Source: CAD feature listing. Evaluate the final solid. Frame: model axes, mm. A direction names the side the tool comes from. Coordinates: 2 decimals unless noted, no trailing zeros. Write each loop counter-clockwise with the first axis right and the second up, starting at its lowest first coordinate (ties: lowest second). Pieces come first, ordered by that corner, then holes. Notation, with made-up numbers: M 20.25,8.5 L 41.25,8.5 A28 ccw 41.25,44.5 Z; hole C 62,-22.5 d6. An arc over 180 degrees is marked long. One line per item, written item: value. Start each with the question number.
Item 1: Cut plane C-C, the plane y = 20. Output: boundary loops of the cut face in (x, z).
Item 2: Set-up query: faces 5 (the flat face through (2.6, 5, 4.9)), 6 (the flat face through (35, 15, 5)), 7 (the cylindrical face through (22.3, 22.5, 5.1)). Return all of +Z, -Z, +X, -X, +Y, -Y with unobstructed straight access to the full face (end or side cutting, diameter ignored); none if empty.
Item 3: Cut plane D-D, the plane x = 26.5. Output: boundary loops of the cut face in (y, z).
Item 4: Mould query, pull axis Z, two halves, no side actions, for faces 1 (the flat face through (10, 16, 5)), 2 (the flat face through (22, 10, 0)), 3 (the cylindrical face through (7, 3, 5)), 4 (the flat face through (22, 10, 10)). Classes: released by +Z, released by -Z, zero draft, split by the parting line, or undercut.
Item 5: Cut plane B-B, the plane z = 5. Output: boundary loops of the cut face in (x, y), then the cut area to 3 significant figures.
Item 6: Ray query, L1, parallel to X at y = 4.5, z = 5.25; L2, parallel to Z at x = 40, y = 1.15; L3, parallel to Y at x = 42, z = 4.25. Return the intervals inside material, ascending. Write a range as from..to.
Item 7: Cut plane A-A, the plane x = 5. Output: boundary loops of the cut face in (y, z).
Item 8: Pin query (flat end, axial travel): P1, Ø4.5, axis at x = 3.5, z = 6.5, coming from the +Y side; P2, Ø2.5, axis at x = 5, z = 5, coming from the +Y side; P3, Ø6, axis at y = 10, z = 6, coming from the -X side. Return the tip coordinate at first contact, or that it passes through.
```python
from build123d import *

# Parameters (mm, degrees)
F1_DEPTH = 10
F3_D     = 5
F5_D     = 4
F6_R     = 0.5
F7_R     = 1


with BuildPart() as f1:
    # F0 (on Top) → F1 (new body)
    with BuildSketch(Plane.XY):
        Polygon((0, 5), (0, 0), (45, 0), (45, 5), (35, 5), (35, 25), (10, 25), (10, 5), align=None)
    extrude(amount=F1_DEPTH)

    # F3 (through all)
    with Locations(Plane.YZ.offset(35)):
        with Locations((20, 5)):
            Hole(F3_D / 2)

    # F5 (through all)
    with Locations(Plane.XZ):
        with Locations((5, 5), (40, 5)):
            Hole(F5_D / 2)

    # F6
    f6_edges = [f1.edges().sort_by_distance(p)[0] for p in [
        (0, 2.5, 10),
        (0, 2.5, 0),
        (45, 2.5, 10),
        (45, 2.5, 0),
    ]]
    fillet(f6_edges, radius=F6_R)

    # F7
    f7_edges = [f1.edges().sort_by_distance(p)[0] for p in [
        (10, 5, 5),
        (35, 5, 5),
    ]]
    fillet(f7_edges, radius=F7_R)


solid = f1.part
```
From the geometry:
1. outline: M 10,0 L 35,0 L 35,2.5 L 10,2.5 Z; M 10,7.5 L 35,7.5 L 35,10 L 10,10 Z
2. face 5: +Z, -Z, -X, +Y
2. face 6: +Z, -Z, +X, +Y
2. face 7: +X, -X
3. outline: M 0,0 L 25,0 L 25,10 L 0,10 Z; hole C 20,5 d5
4. face 1: zero draft
4. face 2: released by -Z
4. face 3: undercut
4. face 4: released by +Z
5. outline: M 0,0 L 3,0 L 3,5 L 0,5 Z; M 7,0 L 38,0 L 38,5 L 36,5 A1 cw 35,6 L 35,17.5 L 10,17.5 L 10,6 A1 cw 9,5 L 7,5 Z; M 10,22.5 L 35,22.5 L 35,25 L 10,25 Z; M 42,0 L 45,0 L 45,5 L 42,5 Z
5. area: 560 mm²
6. L1: x = 0..3.02, 6.98..38.02, 41.98..45
6. L2: z = 0..3, 7..10
6. L3: y = 0..5
7. outline: M 0,0 L 5,0 L 5,3 L 0,3 Z; M 0,7 L 5,7 L 5,10 L 0,10 Z
8. P1: stops at y = 5
8. P2: passes through
8. P3: stops at x = 10
